For this review, take the finished solid that the model builds, in its own axes (mm). Face numbers are marked on the shaded views. A direction names the side the tool comes from. Give positions to 0.01 mm unless a question says otherwise; leave off trailing zeros. Order: outer loops, then holes, each group sorted by start corner. A loop starts at its lowest first (then second) coordinate and runs counter-clockwise, first axis right, second up. Notation, with made-up numbers: M 71.5,54.25 L 126.5,54.25 A16 cw 126.5,74.25 Z; hole C 23,85.5 d7. An arc over 180 degrees is marked long. Answer as CSV lines item,"result". Start each with the question number.
1. Mouldability with a two-part tool opening along Y and no side actions: class the marked faces 1, 2 and 3 as pulls with the +Y half, pulls with the -Y half, needs draft (parallel to the pull), parting line crosses it, or undercut.
2. For line 1 along Y through (x, z) = (0, 3.25) (3 decimals); line 2 along Y through (x, z) = (0, 55.5) (3 decimals); line 3 along Y through (x, z) = (0, 20) (3 decimals), list the stretches that pass through material, from the lowest coordinate up.
3. Clearance check with flat-ended pins moving along their axes: P1, Ø5.5, axis at x = -22.52, y = 13, coming from the +Z side; P2, Ø5, axis at y = 14.5, z = 10, coming from the -X side; P3, Ø10, axis at x = -14, z = 40, coming from the +Y side; P4, Ø2, axis at x = 6.5, z = 39.5, coming from the +Y side. State where each tip first meets the part, or that it passes through.
4. Machinability: for the marked faces 4 and 5, which of the approach directions +Z, -Z, +X, -X, +Y, -Y give a long, thin tool a straight path to every point of the face, cutting with its end or side? Answer none if there is none.
5. We need section B-B, the plane x = 22. Give the boundary of the cut face in (y, z), and give its area (3 significant figures).
6. We need section A-A, the plane y = 0. Give the boundary of the cut face in (x, z) (3 decimals), and give its area (3 significant figures).
7. We need section D-D, the plane z = 27. Give the boundary of the cut face in (x, y) (3 decimals), and give its area (3 significant figures).
8. We need section C-C, the plane z = 5. Give the boundary of the cut face in (x, y) (3 decimals).
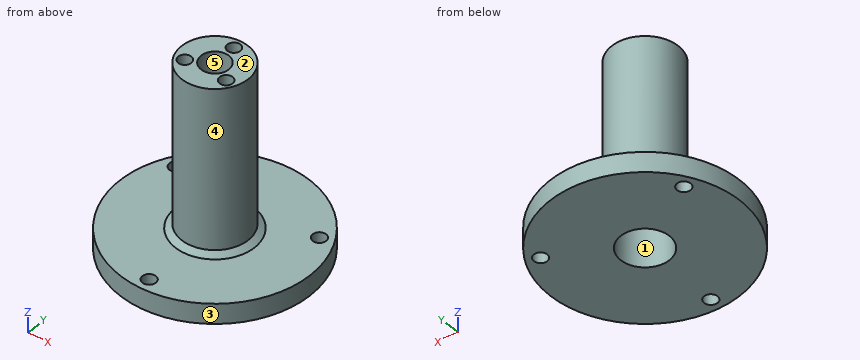
from build123d import *

# Parameters (mm, degrees)
ESQUISSE3_R         = 30
ESQUISSE3_R_2       = 2.125
ESQUISSE3_R_3       = 7.675
BOSS_EXTRU_1_DEPTH  = 6.35
ESQUISSE4_R         = 10.5
ESQUISSE4_R_2       = 7.675
BOSS_EXTRU_2_DEPTH  = 45
SKETCH1_R           = 10.5
SKETCH1_R_2         = 4.375
BOSS_EXTRUDE1_DEPTH = 7
SKETCH2_R           = 2.05
CUT_EXTRUDE1_DEPTH  = 6
CHAMFER2_SIZE       = 5.712592027
CHAMFER2_SIZE_2     = 4
CHAMFER3_SIZE       = 2
CHAMFER3_SIZE2      = 1.349017034


with BuildPart() as part:
    # Esquisse3 → Boss.-Extru.1 (new body)
    with BuildSketch(Plane.XY):
        Circle(ESQUISSE3_R)
        with Locations((-22.516660498, 13)):
            Circle(ESQUISSE3_R_2, mode=Mode.SUBTRACT)
        with Locations((22.516660498, 13)):
            Circle(ESQUISSE3_R_2, mode=Mode.SUBTRACT)
        with Locations((0, -26)):
            Circle(ESQUISSE3_R_2, mode=Mode.SUBTRACT)
        Circle(ESQUISSE3_R_3, mode=Mode.SUBTRACT)
    extrude(amount=BOSS_EXTRU_1_DEPTH)

    # Esquisse4 → Boss.-Extru.2 (add)
    with BuildSketch(Plane.XY.offset(6.35)):
        with Locations(Location((0, 0, 0), (0, 0, 180))):
            Circle(ESQUISSE4_R)
        Circle(ESQUISSE4_R_2, mode=Mode.SUBTRACT)
    extrude(amount=BOSS_EXTRU_2_DEPTH)

    # Sketch1 → Boss-Extrude1 (add)
    with BuildSketch(Plane.XY.offset(51.35)):
        with Locations(Location((0, 0, 0), (0, 0, 180))):
            Circle(SKETCH1_R)
        Circle(SKETCH1_R_2, mode=Mode.SUBTRACT)
    extrude(amount=BOSS_EXTRUDE1_DEPTH)

    # Sketch2 → Cut-Extrude1 (cut)
    with BuildSketch(Plane.XY.offset(58.35)):
        with Locations((0, 7.5)):
            Circle(SKETCH2_R)
        with Locations((-6.495190528, -3.75)):
            Circle(SKETCH2_R)
        with Locations((6.495190528, -3.75)):
            Circle(SKETCH2_R)
    extrude(amount=-CUT_EXTRUDE1_DEPTH, mode=Mode.SUBTRACT)

    # Chamfer2
    # the kernel refuses this chamfer: 5.712592027, 4 mm, written as the material it adds along each edge
    with BuildSketch(Plane(origin=(0, 0, 51.35), x_dir=(1, 0, 0), z_dir=(0, -1, 0))) as chamfer2_piece_1_section:
        Polygon((7.675, -CHAMFER2_SIZE), (7.675 - CHAMFER2_SIZE_2, 0), (7.675, 0), align=None)
    chamfer2_piece_1 = revolve(axis=Axis((0, 0, 51.35), (0, 0, 1)), mode=Mode.PRIVATE)
    chamfer2_piece_1 = chamfer2_piece_1 - Plane(origin=(0, 0, 47.945767055), x_dir=(1, 0, 0), z_dir=(0, 0, -1)) * Cylinder(4.375, 31, mode=Mode.PRIVATE)
    add(chamfer2_piece_1)

    # Chamfer3
    chamfer3_edges = [part.edges().sort_by_distance(p)[0] for p in [
        (10.5, 0, 6.35),
    ]]
    chamfer3_side = [part.faces().sort_by_distance(p)[0] for p in [
        (-29.151471863, 0, 6.35),
    ]]
    chamfer(chamfer3_edges, length=CHAMFER3_SIZE, length2=CHAMFER3_SIZE2, reference=chamfer3_side[0])


solid = part.part
Result set:
1,face 1,"undercut"
1,face 2,"needs draft"
1,face 3,"parting line crosses it"
2,line 1,"-30 to -28.125, -23.875 to -7.675, 7.675 to 30"
2,line 2,"-10.5 to -4.375, 4.375 to 5.45, 9.55 to 10.5"
2,line 3,"-10.5 to -7.675, 7.675 to 10.5"
3,P1,"z = 6.35"
3,P2,"through"
3,P3,"y = 5.41"
3,P4,"y = 8.94"
4,face 4,"+Z"
4,face 5,"+Z, -Z"
5,outline,"M -20.4,0 L 10.94,0 L 10.94,6.35 L -20.4,6.35 Z; M 15.06,0 L 20.4,0 L 20.4,6.35 L 15.06,6.35 Z"
5,area,"233 mm2"
6,outline,"M -30,0 L -7.675,0 L -7.675,45.637 L -4.375,50.35 L -4.375,58.35 L -10.5,58.35 L -10.5,7.699 L -12.5,6.35 L -30,6.35 Z; M 4.375,50.35 L 7.675,45.637 L 7.675,0 L 30,0 L 30,6.35 L 12.5,6.35 L 10.5,7.699 L 10.5,58.35 L 4.375,58.35 Z"
6,area,"648 mm2"
7,outline,"C 0,0 d21; hole C 0,0 d15.35"
7,area,"161 mm2"
8,outline,"C 0,0 d60; hole C -22.517,13 d4.25; hole C 0,0 d15.35; hole C 0,-26 d4.25; hole C 22.517,13 d4.25"
